from build123d import *

# Parameters (mm, degrees)
CROQUIS2_W                                           = 71
CROQUIS2_H                                           = 9.52
SALIENTE_EXTRUIR1_DEPTH                              = 60
CROQUIS3_R                                           = 2.38
CORTAR_EXTRUIR1_DEPTH                                = 15
CORTAR_EXTRUIR2_REACH                                = 95.443
REFRENTADO_PARA_TORNILLO_TAP_N_CON_CABEZ_D           = 4.3
REFRENTADO_PARA_TORNILLO_TAP_N_CON_CABEZ_DEPTH       = 17
REFRENTADO_PARA_TORNILLO_TAP_N_CON_CABEZ_CBORE_D     = 7.5
REFRENTADO_PARA_TORNILLO_TAP_N_CON_CABEZ_CBORE_DEPTH = 4
REFRENTADO_PARA_TORNILLO_TAP_N_CON_CABEZ_TIP         = 1.291850331


with BuildPart() as part:
    # Croquis2 → Saliente-Extruir1 (new body)
    with BuildSketch(Plane.XY):
        with Locations((35.5, 4.76)):
            Rectangle(CROQUIS2_W, CROQUIS2_H)
    extrude(amount=SALIENTE_EXTRUIR1_DEPTH)

    # Croquis3 → Cortar-Extruir1 (cut)
    with BuildSketch(Plane(origin=(0, 0, 0), x_dir=(-1, 0, 0), z_dir=(0, 0, -1))):
        with Locations((-54, 4.74)):
            Circle(CROQUIS3_R)
        with Locations((-18, 4.74)):
            Circle(CROQUIS3_R)
    extrude(amount=-CORTAR_EXTRUIR1_DEPTH, mode=Mode.SUBTRACT)

    # Croquis4 → Cortar-Extruir2 (cut, up to next)
    with BuildSketch(Plane(origin=(0, 9.52, 0), x_dir=(1, 0, 0), z_dir=(0, 1, 0)), mode=Mode.PRIVATE) as cortar_extruir2_sk1:
        with BuildLine():
            Line((61, -5), (66, -5))
            ThreePointArc((66, -5), (69, -8), (66, -11))
            Line((66, -11), (61, -11))
            ThreePointArc((61, -11), (58, -8), (61, -5))
        make_face()
    cortar_extruir2_tool1 = extrude(cortar_extruir2_sk1.sketch, amount=-CORTAR_EXTRUIR2_REACH, mode=Mode.PRIVATE) & part.part
    # Croquis4 → Cortar-Extruir2 (cut, up to next)
    with BuildSketch(Plane(origin=(0, 9.52, 0), x_dir=(1, 0, 0), z_dir=(0, 1, 0)), mode=Mode.PRIVATE) as cortar_extruir2_sk2:
        with BuildLine():
            Line((61, -49), (66, -49))
            ThreePointArc((66, -49), (69, -52), (66, -55))
            Line((66, -55), (61, -55))
            ThreePointArc((61, -55), (58, -52), (61, -49))
        make_face()
    cortar_extruir2_tool2 = extrude(cortar_extruir2_sk2.sketch, amount=-CORTAR_EXTRUIR2_REACH, mode=Mode.PRIVATE) & part.part
    # Croquis4 → Cortar-Extruir2 (cut, up to next)
    with BuildSketch(Plane(origin=(0, 9.52, 0), x_dir=(1, 0, 0), z_dir=(0, 1, 0)), mode=Mode.PRIVATE) as cortar_extruir2_sk3:
        with BuildLine():
            Line((5, -5), (10, -5))
            ThreePointArc((10, -5), (13, -8), (10, -11))
            Line((10, -11), (5, -11))
            ThreePointArc((5, -11), (2, -8), (5, -5))
        make_face()
    cortar_extruir2_tool3 = extrude(cortar_extruir2_sk3.sketch, amount=-CORTAR_EXTRUIR2_REACH, mode=Mode.PRIVATE) & part.part
    # Croquis4 → Cortar-Extruir2 (cut, up to next)
    with BuildSketch(Plane(origin=(0, 9.52, 0), x_dir=(1, 0, 0), z_dir=(0, 1, 0)), mode=Mode.PRIVATE) as cortar_extruir2_sk4:
        with BuildLine():
            Line((5, -49), (10, -49))
            ThreePointArc((10, -49), (13, -52), (10, -55))
            Line((10, -55), (5, -55))
            ThreePointArc((5, -55), (2, -52), (5, -49))
        make_face()
    cortar_extruir2_tool4 = extrude(cortar_extruir2_sk4.sketch, amount=-CORTAR_EXTRUIR2_REACH, mode=Mode.PRIVATE) & part.part
    add(cortar_extruir2_tool1.solids().sort_by_distance((63.5, 9.52, 8))[0], mode=Mode.SUBTRACT)
    add(cortar_extruir2_tool2.solids().sort_by_distance((63.5, 9.52, 52))[0], mode=Mode.SUBTRACT)
    add(cortar_extruir2_tool3.solids().sort_by_distance((7.5, 9.52, 8))[0], mode=Mode.SUBTRACT)
    add(cortar_extruir2_tool4.solids().sort_by_distance((7.5, 9.52, 52))[0], mode=Mode.SUBTRACT)

    # Refrentado para tornillo tapón con cabeza de clavija de M41
    with Locations(Plane(origin=(0, 0, 0), x_dir=(-1, 0, 0), z_dir=(0, -1, 0))):
        with Locations((-50.5, -35), (-50.5, -55), (-20.5, -55), (-20.5, -35)):
            CounterBoreHole(REFRENTADO_PARA_TORNILLO_TAP_N_CON_CABEZ_D / 2, REFRENTADO_PARA_TORNILLO_TAP_N_CON_CABEZ_CBORE_D / 2, REFRENTADO_PARA_TORNILLO_TAP_N_CON_CABEZ_CBORE_DEPTH, depth=REFRENTADO_PARA_TORNILLO_TAP_N_CON_CABEZ_DEPTH)
            with Locations((0, 0, -(REFRENTADO_PARA_TORNILLO_TAP_N_CON_CABEZ_DEPTH + REFRENTADO_PARA_TORNILLO_TAP_N_CON_CABEZ_TIP / 2))):  # 118° drill point
                Cone(0, REFRENTADO_PARA_TORNILLO_TAP_N_CON_CABEZ_D / 2, REFRENTADO_PARA_TORNILLO_TAP_N_CON_CABEZ_TIP, mode=Mode.SUBTRACT)


solid = part.part
Work out the finished part from the listing and answer in its coordinate system (mm). A direction names the side the tool comes from. Round coordinates to 2 decimals unless told otherwise and drop trailing zeros. Write each loop counter-clockwise with the first axis right and the second up, starting at its lowest first coordinate (ties: lowest second). Pieces come first, ordered by that corner, then holes. Notation, with made-up numbers: M 1.5,-28 L 33.5,-28 A30 cw 33.5,-6 Z; hole C 29.25,32 d2. An arc over 180 degrees is marked long. Use a Markdown table: item, result.
1) The part is cut by section A-A on z = 52. Give the vertices of the cut face in (x, y), plus the area to 3 significant figures.
Taken from the geometry:
| item | result |
|---|---|
| outline | M 0,0 L 2,0 L 2,9.52 L 0,9.52 Z; M 13,0 L 18.25,0 L 18.25,4 L 22.75,4 L 22.75,0 L 48.25,0 L 48.25,4 L 52.75,4 L 52.75,0 L 58,0 L 58,9.52 L 13,9.52 Z; M 69,0 L 71,0 L 71,9.52 L 69,9.52 Z |
| area | 430 mm2 |
2) Determine the mould class of faces 6 (the face through (35, 9.52, 30)), 7 (the face through (19, 4, 57)), 8 (the face through (18, 5, 15)), 9 (the face through (64, 5, 55)) for opening direction Z: pulls with the +Z half, pulls with the -Z half, needs draft (parallel to the pull), parting line crosses it, or undercut.
Taken from the geometry:
| item | result |
|---|---|
| face 6 | needs draft |
| face 7 | undercut |
| face 8 | pulls with the -Z half |
| face 9 | undercut |
3) A flat-ended cylindrical pin translates along its axis: pin 1 (1.4 mm diameter, centred on x = 53, y = 5.5, fed in from -Z). Find the tip coordinate at first contact, or state that the pin passes through.
Taken from the geometry:
| item | result |
|---|---|
| pin 1 | stops at z = 15 |
4) The part is cut by section C-C on y = 8. State how many separate pieces and enclosed holes the cut face has, plus the area to 3 significant figures.
Taken from the geometry:
| item | result |
|---|---|
| separate pieces | 1 |
| enclosed holes | 8 |
| area | 3,970 mm2 |
5) The part is cut by section B-B on x = 50.5. Give the vertices of the cut face in (y, z).
Taken from the geometry:
| item | result |
|---|---|
| outline | M 0,0 L 9.52,0 L 9.52,32.85 L 4,32.85 L 4,31.25 L 0,31.25 Z; M 0,38.75 L 4,38.75 L 4,37.15 L 9.52,37.15 L 9.52,52.85 L 4,52.85 L 4,51.25 L 0,51.25 Z; M 0,58.75 L 4,58.75 L 4,57.15 L 9.52,57.15 L 9.52,60 L 0,60 Z |
6) The part is cut by section D-D on z = 10. Give the vertices of the cut face in (x, y), plus the area to 3 significant figures.
Taken from the geometry:
| item | result |
|---|---|
| outline | M 0,0 L 2.76,0 L 2.76,9.52 L 0,9.52 Z; M 12.24,0 L 58.76,0 L 58.76,9.52 L 12.24,9.52 Z; M 68.24,0 L 71,0 L 71,9.52 L 68.24,9.52 Z; hole C 18,4.74 d4.76; hole C 54,4.74 d4.76 |
| area | 460 mm2 |
7) Consider line 1 (Z direction, x = 50.5, y = 2.15); line 2 (Z direction, x = 61.5, y = 4); line 3 (X direction, y = 7.25, z = 35). Determine where each line is inside the solid, lowest interval first. Write a range as [from, to].
Taken from the geometry:
| item | result |
|---|---|
| line 1 | z = [0, 31.25], [38.75, 51.25], [58.75, 60] |
| line 2 | z = [0, 5], [11, 49], [55, 60] |
| line 3 | x = [0, 18.35], [22.65, 48.35], [52.65, 71] |
8) Which of the six approach directions +Z, -Z, +X, -X, +Y, -Y give full straight-line access (tool end or side, diameter ignored) to faces 1 (the face through (49, 4, 57)), 2 (the face through (2, 5, 52)), 3 (the face through (0, 5, 30)), 4 (the face through (56.378, 4.845, 7.395)), 5 (the face through (35, 5, 60))?
Taken from the geometry:
| item | result |
|---|---|
| face 1 | -Y |
| face 2 | +Y, -Y |
| face 3 | +Z, -Z, -X, +Y, -Y |
| face 4 | -Z |
| face 5 | +Z, +X, -X, +Y, -Y |
